Source: three-view drawing plus pictorial views. Frame: mm from the lowest corner of the part. A direction names the side the tool comes from. Coordinates: 2 decimals unless noted, no trailing zeros. Write each loop counter-clockwise with the first axis right and the second up, starting at its lowest first coordinate (ties: lowest second). Pieces come first, ordered by that corner, then holes. Notation, with made-up numbers: (-3, -25.75) - (33, -25.75) arc R15 cw to (33, -14.75) - close; hole circle Ø6 at (40, 77.5). An arc over 180 degrees is marked (long way). Put each result on its own line as item: value. Start each with the question number.
1. Line query: line 1 (Z direction, x = 4, y = 1.5); line 2 (X direction, y = 8.5, z = 6); line 3 (X direction, y = 2.25, z = 6.5) (1 decimal). Output: solid intervals per line, ascending.
2. Cut plane A-A, the plane y = 14. Return loops of the section in (x, z) (1 decimal).
3. Access query for the marked faces 4 and 5. Directions: +Z, -Z, +X, -X, +Y, -Y. A direction counts if a zero-diameter tool reaches every point of the face in a straight line with its end or side. Return the directions, or none.
4. Pin query (flat end, axial travel): pin 1 (1.5 mm diameter, centred on y = 13, z = 6.5, fed in from +X); pin 2 (1.6 mm diameter, centred on x = 4.58, z = 3.97, fed in from +Y) (1 decimal). Return the tip coordinate at first contact, or that it passes through.
5. Pull-direction query (X, two-part tool) for the marked faces 1, 2 and 3; classes: released by +X, released by -X, zero draft, split by the parting line, or undercut.
6. Cut plane B-B, the plane y = 8. Return loops of the section in (x, z) (1 decimal).
7. Cut plane D-D, the plane z = 2. Return loops of the section in (x, y) (1 decimal).
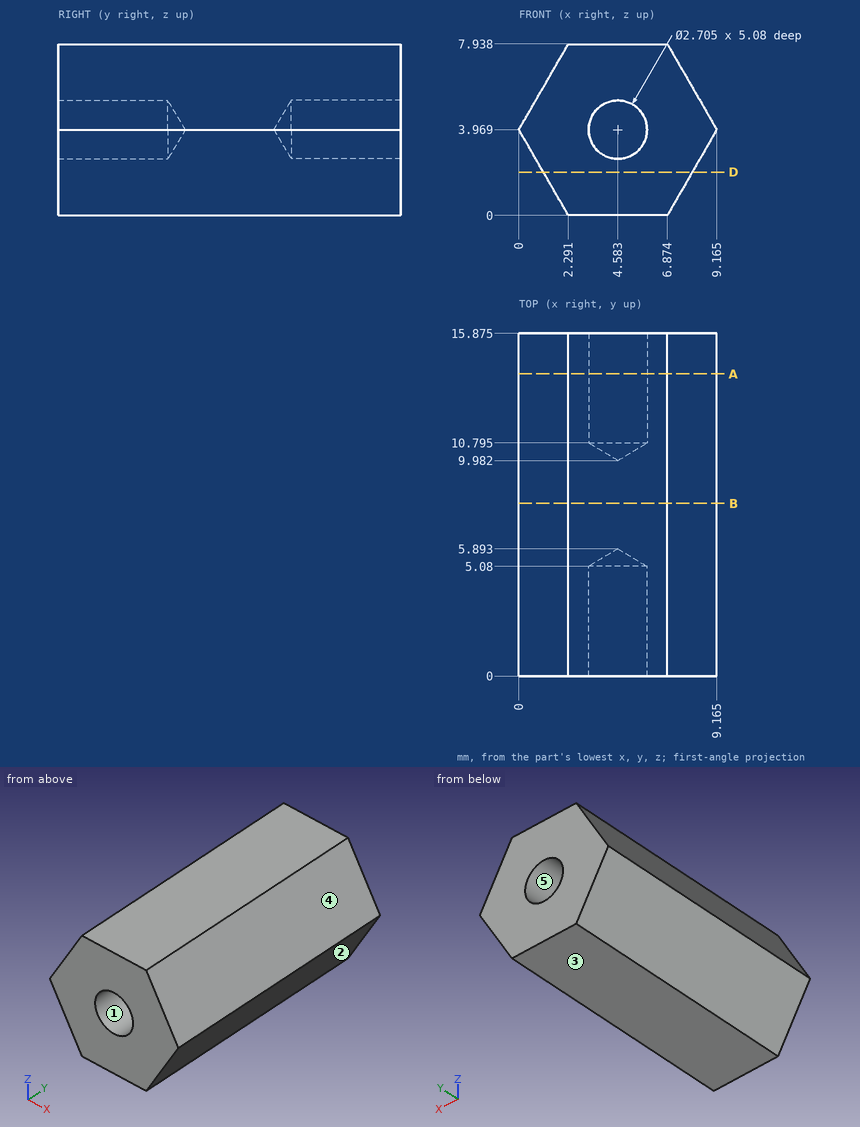
Report:
1. line 1: z = 0 to 2.75, 5.19 to 7.94
1. line 2: x = 1.17 to 7.99
1. line 3: x = 1.5 to 7.7
2. outline: (0, 4) - (2.3, 0) - (6.9, 0) - (9.2, 4) - (6.9, 7.9) - (2.3, 7.9) - close; hole circle Ø2.7 at (4.6, 4)
3. face 4: +Z, +X, +Y, -Y
3. face 5: +Y
4. pin 1: stops at x = 8.14
4. pin 2: stops at y = 10.5
5. face 1: undercut
5. face 2: released by +X
5. face 3: zero draft
6. outline: (0, 4) - (2.3, 0) - (6.9, 0) - (9.2, 4) - (6.9, 7.9) - (2.3, 7.9) - close
7. outline: (1.1, 0) - (8, 0) - (8, 15.9) - (1.1, 15.9) - close
